from build123d import *

# Parameters (mm, degrees)
F1_R     = 1.5
F1_W     = 23.025
F1_H     = 42.14
F2_DEPTH = 3
F4_DEPTH = 23.025
F6_DEPTH = 23.025
F8_DEPTH = 2


with BuildPart() as f2:
    # F1 (on Top) → F2 (new body)
    with BuildSketch(Plane.XY):
        with BuildLine():
            ThreePointArc((4, 48.44), (1.383705, 47.356295), (0.3, 44.74))
            Line((0.3, 44.74), (0.3, 0))
            ThreePointArc((0.3, 0), (1.383705, -2.616295), (4, -3.7))
            Line((4, -3.7), (70.35, -3.7))
            Line((70.35, -3.7), (70.35, 44.74))
            ThreePointArc((70.35, 44.74), (69.266295, 47.356295), (66.65, 48.44))
            Line((66.65, 48.44), (4, 48.44))
        make_face()
        with Locations((4, 0)):
            Circle(F1_R, mode=Mode.SUBTRACT)
        with Locations((19.8125, 22.37)):
            Rectangle(F1_W, F1_H, mode=Mode.SUBTRACT)
        with Locations((4, 44.74)):
            Circle(F1_R, mode=Mode.SUBTRACT)
        with Locations((50.8375, 22.37)):
            Rectangle(F1_W, F1_H, mode=Mode.SUBTRACT)
        with Locations((66.65, 44.74)):
            Circle(F1_R, mode=Mode.SUBTRACT)
    extrude(amount=F2_DEPTH)

    # F3 (on face) → F4 (join)
    with BuildSketch(Plane(origin=(31.325, 0, 0), x_dir=(0, -1, 0), z_dir=(-1, 0, 0))):
        Polygon((-22.774145, 3), (-23.697906, 3), (-21.965855, 0), (-21.042094, 0), align=None)
        Polygon((-19.829659, 3), (-20.753419, 3), (-19.021368, 0), (-18.097608, 0), align=None)
        Polygon((-16.885172, 3), (-17.808933, 3), (-16.076882, 0), (-15.153122, 0), align=None)
        Polygon((-13.940686, 3), (-14.864447, 3), (-13.132396, 0), (-12.208635, 0), align=None)
        Polygon((-10.9962, 3), (-11.91996, 3), (-10.187909, 0), (-9.264149, 0), align=None)
        Polygon((-8.051713, 3), (-8.975474, 3), (-7.243423, 0), (-6.319663, 0), align=None)
        Polygon((-5.107227, 3), (-6.030987, 3), (-4.298937, 0), (-3.375176, 0), align=None)
        Polygon((-3.086501, 3), (-1.35445, 0), (-1.3, 0), (-1.3, 1.505689), (-2.162741, 3), align=None)
        Polygon((-23.986581, 0), (-25.718632, 3), (-26.642392, 3), (-24.910341, 0), align=None)
        Polygon((-26.931067, 0), (-28.663118, 3), (-29.586878, 3), (-27.854828, 0), align=None)
        Polygon((-29.875553, 0), (-31.607604, 3), (-32.531365, 3), (-30.799314, 0), align=None)
        Polygon((-32.82004, 0), (-34.552091, 3), (-35.475851, 3), (-33.7438, 0), align=None)
        Polygon((-37.496577, 3), (-38.420337, 3), (-36.688287, 0), (-35.764526, 0), align=None)
        Polygon((-38.709013, 0), (-40.441063, 3), (-41.364824, 3), (-39.632773, 0), align=None)
        Polygon((-42.577259, 0), (-41.653499, 0), (-43.38555, 3), (-43.44, 3), (-43.44, 1.494311), align=None)
    extrude(amount=F4_DEPTH)

    # F5 (on face) → F6 (join)
    with BuildSketch(Plane.YZ.offset(39.325)):
        Polygon((23.697906, 3), (22.774145, 3), (21.042094, 0), (21.965855, 0), align=None)
        Polygon((26.642392, 3), (25.718632, 3), (23.986581, 0), (24.910341, 0), align=None)
        Polygon((29.586878, 3), (28.663118, 3), (26.931067, 0), (27.854828, 0), align=None)
        Polygon((32.531365, 3), (31.607604, 3), (29.875553, 0), (30.799314, 0), align=None)
        Polygon((35.475851, 3), (34.552091, 3), (32.82004, 0), (33.7438, 0), align=None)
        Polygon((38.420337, 3), (37.496577, 3), (35.764526, 0), (36.688287, 0), align=None)
        Polygon((41.364824, 3), (40.441063, 3), (38.709013, 0), (39.632773, 0), align=None)
        Polygon((43.44, 1.494311), (43.44, 3), (43.38555, 3), (41.653499, 0), (42.577259, 0), align=None)
        Polygon((19.021368, 0), (20.753419, 3), (19.829659, 3), (18.097608, 0), align=None)
        Polygon((16.076882, 0), (17.808933, 3), (16.885172, 3), (15.153122, 0), align=None)
        Polygon((13.132396, 0), (14.864447, 3), (13.940686, 3), (12.208635, 0), align=None)
        Polygon((10.187909, 0), (11.91996, 3), (10.9962, 3), (9.264149, 0), align=None)
        Polygon((7.243423, 0), (8.975474, 3), (8.051713, 3), (6.319663, 0), align=None)
        Polygon((4.298937, 0), (6.030987, 3), (5.107227, 3), (3.375176, 0), align=None)
        Polygon((1.3, 1.505689), (1.3, 0), (1.35445, 0), (3.086501, 3), (2.162741, 3), align=None)
    extrude(amount=F6_DEPTH)

    # F7 (on face) → F8 (cut)
    with BuildSketch(Plane(origin=(0, 0, 0), x_dir=(1, 0, 0), z_dir=(0, 0, -1))):
        with BuildLine():
            Line((7.3, 0), (7.3, 3.7))
            Line((7.3, 3.7), (4, 3.7))
            ThreePointArc((4, 3.7), (1.383705, 2.616295), (0.3, 0))
            Line((0.3, 0), (0.3, -3.3))
            Line((0.3, -3.3), (4, -3.3))
            ThreePointArc((4, -3.3), (6.333452, -2.333452), (7.3, 0))
        make_face()
        with BuildLine():
            Line((0.3, -41.44), (0.3, -44.74))
            ThreePointArc((0.3, -44.74), (1.383705, -47.356295), (4, -48.44))
            Line((4, -48.44), (7.3, -48.44))
            Line((7.3, -48.44), (7.3, -44.74))
            ThreePointArc((7.3, -44.74), (6.333452, -42.406548), (4, -41.44))
            Line((4, -41.44), (0.3, -41.44))
        make_face()
        with BuildLine():
            Line((63.35, -48.44), (66.65, -48.44))
            ThreePointArc((66.65, -48.44), (69.266295, -47.356295), (70.35, -44.74))
            Line((70.35, -44.74), (70.35, -41.44))
            Line((70.35, -41.44), (66.65, -41.44))
            ThreePointArc((66.65, -41.44), (64.316548, -42.406548), (63.35, -44.74))
            Line((63.35, -44.74), (63.35, -48.44))
        make_face()
    extrude(amount=-F8_DEPTH, mode=Mode.SUBTRACT)


solid = f2.part
Source: CAD feature listing. Evaluate the final solid. Frame: model axes, mm. A direction names the side the tool comes from. Round coordinates to 2 decimals unless told otherwise and drop trailing zeros. Use a Markdown table: item, result. Add a question column.
1. Line query: probe 1 along X at (y, z) = (43, 2.85) (3 decimals); probe 2 along Y at (x, z) = (4, 2.3); probe 3 along X at (y, z) = (44.74, 2.55). Output: solid intervals per line, ascending.
2. Mould query, pull axis Y, two halves, no side actions, for faces 5 (the flat face through (2, 3.3, 1)), 6 (the flat face through (19.974, 16.955, 1.521)), 7 (the flat face through (69, 41.44, 1)). Classes: +Y half, -Y half, draft (parallel to the pull), parting line (faces both ways), or undercut.
3. Section query A-A (x = 46.5). Give the number of separate pieces and of enclosed holes in the cut face, then the cut area to 3 significant figures.
4. Set-up query: faces 1 (the flat face through (50.68, 36.64, 1.52)), 2 (the flat face through (8.3, 33, 1)), 3 (the cylindrical face through (1.41, 47.38, 2.49)), 4 (the flat face through (20, 40.5, 1.5)). Return all of +Z, -Z, +X, -X, +Y, -Y with unobstructed straight access to the full face (end or side cutting, diameter ignored); none if empty.
5. First-contact query: pin 1 (2.5 mm diameter, centred on x = 4, y = 44.74, fed in from -Z). Flat tip, straight axial feed; report the tip coordinate or a pass-through.
Derived:
| question | item | result |
|---|---|---|
| 1 | probe 1 | 0.3 to 8.3, 31.325 to 39.325, 62.35 to 70.35 |
| 1 | probe 2 | -3.7 to -1.5, 1.5 to 43.24, 46.24 to 48.44 |
| 1 | probe 3 | 0.3 to 2.5, 5.5 to 65.15, 68.15 to 70.35 |
| 2 | face 5 | -Y half |
| 2 | face 6 | undercut |
| 2 | face 7 | +Y half |
| 3 | separate pieces | 15 |
| 3 | enclosed holes | 0 |
| 3 | area | 70.3 mm2 |
| 4 | face 1 | +Z |
| 4 | face 2 | none |
| 4 | face 3 | +Z, -Z, -X, +Y |
| 4 | face 4 | -Z |
| 5 | pin 1 | through |
